Verification items for the finished model (mm, model axes). A direction names the side the tool comes from. Round coordinates to 2 decimals unless told otherwise and drop trailing zeros. Order: outer loops, then holes, each group sorted by start corner. A loop starts at its lowest first (then second) coordinate and runs counter-clockwise, first axis right, second up. Notation, with made-up numbers: (-1.75, 76.25) -> (33.25, 76.25) arc R31 cw to (33.25, 103.25) -> close; hole circle Ø1 at (41, 56.5). An arc over 180 degrees is marked (long way). Return JSON: item names as keys, results as strings. Group by question number.
Item 1: Depth check by flat-ended pin: pin 1 Ø5 at (x, z) = (6, 3) entering from +Y; pin 2 Ø1 at (x, z) = (-2, 0) entering from +Y; pin 3 Ø3 at (x, z) = (-5.5, -3) entering from -Y. Enter the tip coordinate at first touch or a pass-through.
Item 2: Scan lines: probe 1 along X at (y, z) = (2.75, 2.5); probe 2 along Y at (x, z) = (-1, 0); probe 3 along X at (y, z) = (1, 1.25). Record each from-to range of solid material in increasing order. Write a range as from..to.
Item 3: Sectioned sample at C-C on y = 0.5. Record the cut outline in (x, z).
Item 4: Sectioned sample at B-B on x = -2. Record the cut outline in (y, z).
Item 5: Sectioned sample at A-A on z = 0. Record the cut outline in (x, y), plus the area to 4 significant figures.
Item 6: Sectioned sample at D-D on z = -3.5. Record the cut outline in (x, y), plus the area to 3 significant figures.
Item 7: Draft check along Z on faces 3 (the cylindrical face through (2.75, 2.44, -0.54)), 4 (the flat face through (-15, -2, 2)), 5 (the flat face through (-19, -2, 0)). Enter one of: pulls with the +Z half, pulls with the -Z half, needs draft (parallel to the pull), parting line crosses it, or undercut.
Item 8: Access from +Z, -Z, +X, -X, +Y, -Y to the whole of each face (thin tool, end or side, straight path). Record for faces 1 (the cylindrical face through (-17.465, -3.584, 2.285)), 2 (the flat face through (-19, 2, 0)).
Solid Edge part; units mm, degrees
sketch "Sketch1" plane through (10.8674, 0, 10.8674) normal (0, -1, 0) x (1, 0, 0)
  line L0 (-30.8674, -10.8674) -> (-30.8674, -6.6174)
  line L1 (-30.8674, -6.6174) -> (-25.8674, -6.6174)
  line L2 (-25.8674, -6.6174) -> (-25.8674, -8.3674)
  line L3 (-25.8674, -8.3674) -> (9.1326, -8.3674)
  line L4 (9.1326, -8.3674) -> (9.1326, -10.8674)
revolve "RevolvedProtrusion1" add sketch "Sketch1" angle 360 about axis through (16.5, 0, 0) along (-1, 0, 0)
sketch "Sketch2" plane through (-20, 0, 0) normal (-1, 0, 0) x (0, 0, -1)
  line L0 (2.3094, 0) -> (1.1547, 2)
  line L1 (1.1547, 2) -> (-1.1547, 2)
  line L2 (-1.1547, 2) -> (-2.3094, 0)
  line L3 (-2.3094, 0) -> (-1.1547, -2)
  line L4 (-1.1547, -2) -> (1.1547, -2)
  line L5 (1.1547, -2) -> (2.3094, 0)
extrude "Cutout1" cut sketch "Sketch2" against normal blind 2.5
cosmetic_thread "Thread1"
properties material "Steel"
Recorded:
{
 "1": {"pin 1": "y = 2.45", "pin 2": "y = 2.5", "pin 3": "y = -2"},
 "2": {"probe 1": "-20..-15", "probe 2": "-2.5..2.5", "probe 3": "-17.5..20"},
 "3": {"outline": "(-20, -4.22) -> (-15, -4.22) -> (-15, -2.45) -> (20, -2.45) -> (20, 2.45) -> (-15, 2.45) -> (-15, 4.22) -> (-20, 4.22) -> (-20, 2.02) -> (-17.5, 2.02) -> (-17.5, -2.02) -> (-20, -2.02) -> close"},
 "4": {"outline": "circle Ø5 at (0, 0)"},
 "5": {"outline": "(-20, -4.25) -> (-15, -4.25) -> (-15, -2.5) -> (20, -2.5) -> (20, 2.5) -> (-15, 2.5) -> (-15, 4.25) -> (-20, 4.25) -> (-20, 2) -> (-17.5, 2) -> (-17.5, -2) -> (-20, -2) -> close", "area": "207.5 mm²"},
 "6": {"outline": "(-20, -2.41) -> (-15, -2.41) -> (-15, 2.41) -> (-20, 2.41) -> close", "area": "24.1 mm²"},
 "7": {"face 3": "parting line crosses it", "face 4": "needs draft", "face 5": "undercut"},
 "8": {"face 1": "+X, -X", "face 2": "-X"}
}
